```python
from build123d import *

# Parameters (mm, degrees)
F1_DEPTH = 400
F2_R     = 77
F3_DEPTH = 295.001
F4_R     = 100


with BuildPart() as f1:
    # F0 (on Front) → F1 (new body)
    with BuildSketch(Plane.XZ):
        Polygon((69.759124, 160.54423), (-235.240876, 160.54423), (-235.240876, -134.45577), (244.759124, -134.45577), (244.759124, 565.54423), (69.759124, 565.54423), align=None)
    extrude(amount=F1_DEPTH)

    # F2 (on face) → F3 (cut, through all)
    with BuildSketch(Plane.XY.offset(160.54423)):
        with Locations((-82.240876, -202)):
            Circle(F2_R)
    extrude(amount=-F3_DEPTH, mode=Mode.SUBTRACT)

    # F4
    f4_edges = [f1.edges().sort_by_distance(p)[0] for p in [
        (-235.240876, 0, 13.04423),
        (-235.240876, -400, 13.04423),
        (244.759124, -400, 215.54423),
        (244.759124, 0, 215.54423),
    ]]
    fillet(f4_edges, radius=F4_R)


solid = f1.part
```
The listing builds one solid part. Answer for the finished solid, in the listing's coordinates (mm). A direction names the side the tool comes from. Round coordinates to 2 decimals unless told otherwise and drop trailing zeros. Write each loop counter-clockwise with the first axis right and the second up, starting at its lowest first coordinate (ties: lowest second). Pieces come first, ordered by that corner, then holes. Notation, with made-up numbers: (16, 1) -> (36, 1) arc R23 cw to (36, 9) -> close; hole circle Ø7 at (81.25, 75.5). An arc over 180 degrees is marked (long way). Use CSV: the item, a comma, the result in double quotes. Start each with the question number.
(1) Which of the six approach directions +Z, -Z, +X, -X, +Y, -Y give full straight-line access (tool end or side, diameter ignored) to faces 1 (the face through (-13, -153, 160.544)), 2 (the face through (214.69, -371.48, 220.44))?
(2) Consider L1, parallel to Z at x = 62, y = -374.5; L2, parallel to X at y = -169, z = 214; L3, parallel to Y at x = -75, z = 145. Determine where each line is inside the solid, lowest interval first. Write a range as from..to.
(3) Section C-C on x = -20 is taken. Give the vertices of the cut face in (y, z), then the cut area to 3 significant figures.
(4) Each of these flat-tipped pins is pushed along its axis until it touches: pin 1 (1 mm diameter, centred on y = -80.5, z = -53, fed in from +X); pin 2 (2 mm diameter, centred on x = -181.5, z = 147.5, fed in from +Y); pin 3 (1.5 mm diameter, centred on y = -50.5, z = 276, fed in from +X). Where does it stop, or does it pass through?
(5) The mould has two halves that part along X. Classify faces 3 (the face through (1, -197, -134.456)), 4 (the face through (214.69, -28.52, 220.44)), 5 (the face through (69.759, -197, 366)), 6 (the face through (-98.93, -277.17, 15.11)): released by +X, released by -X, zero draft, split by the parting line, or undercut.
(6) Section D-D on y = -149.5 is taken. Give the vertices of the cut face in (x, z).
(7) Section A-A on y = -202 is taken. Give the vertices of the cut face in (x, z).
(8) Section B-B on z = 117.5 is taken. Give the vertices of the cut face in (x, y).
A:
1,face 1,"+Z, -X, +Y, -Y"
1,face 2,"+Z, -Z, +X, -Y"
2,L1,"z = -134.46..160.54"
2,L2,"x = 69.76..244.76"
2,L3,"y = -400..-278.66, -125.34..0"
3,outline,"(-400, -134.46) -> (-247.33, -134.46) -> (-247.33, 160.54) -> (-400, 160.54) -> close; (-156.67, -134.46) -> (0, -134.46) -> (0, 160.54) -> (-156.67, 160.54) -> close"
3,area,"91,300 mm²"
4,pin 1,"stops at x = 242.94"
4,pin 2,"stops at y = -10.83"
4,pin 3,"stops at x = 232.07"
5,face 3,"zero draft"
5,face 4,"released by +X"
5,face 5,"released by -X"
5,face 6,"undercut"
6,outline,"(-235.24, -134.46) -> (-138.57, -134.46) -> (-138.57, 160.54) -> (-235.24, 160.54) -> close; (-25.91, -134.46) -> (244.76, -134.46) -> (244.76, 565.54) -> (69.76, 565.54) -> (69.76, 160.54) -> (-25.91, 160.54) -> close"
7,outline,"(-235.24, -134.46) -> (-159.24, -134.46) -> (-159.24, 160.54) -> (-235.24, 160.54) -> close; (-5.24, -134.46) -> (244.76, -134.46) -> (244.76, 565.54) -> (69.76, 565.54) -> (69.76, 160.54) -> (-5.24, 160.54) -> close"
8,outline,"(-235.24, -300) arc R100 ccw to (-135.24, -400) -> (144.76, -400) arc R100 ccw to (244.76, -300) -> (244.76, -100) arc R100 ccw to (144.76, 0) -> (-135.24, 0) arc R100 ccw to (-235.24, -100) -> close; hole circle Ø154 at (-82.24, -202)"
